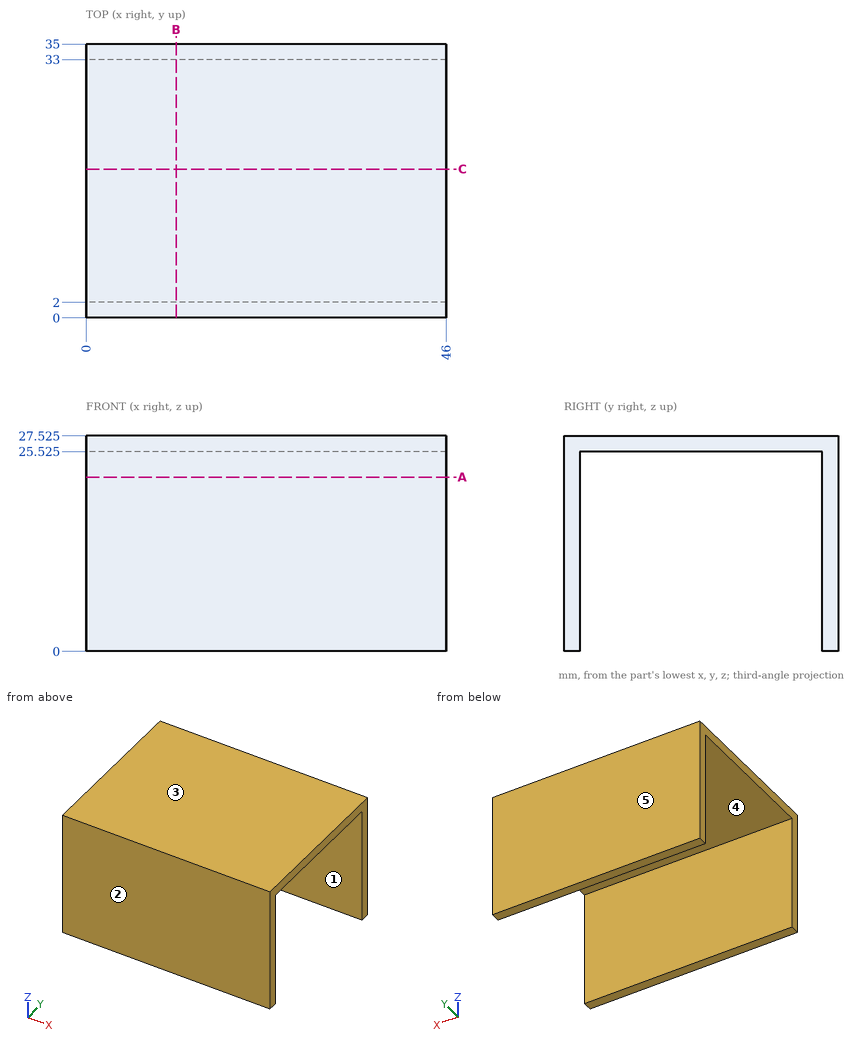
Job drawing, mm, ordinate dimensions from the low corner. One solid piece. A direction names the side the tool comes from. Give positions to 0.01 mm unless a question says otherwise; leave off trailing zeros. Write each loop counter-clockwise with the first axis right and the second up, starting at its lowest first coordinate (ties: lowest second). Pieces come first, ordered by that corner, then holes. Notation, with made-up numbers: M 50.25,51.5 L 93.25,51.5 A13 cw 93.25,71.5 Z; hole C 82.5,-25 d5. An arc over 180 degrees is marked long. One line per item, written item: value. Start each with the question number.
Q1. Probe probe 1 along Y at (x, z) = (15.5, 16); probe 2 along Z at (x, y) = (41, 19) (1 decimal). List the from-to ranges inside material, lowest first. Write a range as [from, to].
Q2. Saw through at C-C, the plane y = 19. Write the cut outline in (x, z) (1 decimal), plus the area to 3 significant figures.
Q3. Saw through at B-B, the plane x = 11.5. Write the cut outline in (y, z) (1 decimal), plus the area to 3 significant figures.
Q4. Two-plate mould, pull along Y, no slides. Class the marked faces 1, 2 and 3: +Y half, -Y half, draft (parallel to the pull), parting line (faces both ways), or undercut.
Q5. Saw through at A-A, the plane z = 22.25. Write the cut outline in (x, y), plus the area to 3 significant figures.
Q6. Drop a flat-ended pin along its axis: pin 1 Ø15.5 at (x, y) = (30.5, 24.5) entering from -Z (1 decimal). Give the stop position or say it passes through.
Q7. 3-axis set-ups, long thin cutter, end or side, ignore diameter. For the marked faces 4 and 5: which of +Z, -Z, +X, -X, +Y, -Y reach the whole face in a straight line?
Output values:
1. probe 1: y = [0, 2], [33, 35]
1. probe 2: z = [25.5, 27.5]
2. outline: M 0,25.5 L 46,25.5 L 46,27.5 L 0,27.5 Z
2. area: 92.0 mm²
3. outline: M 0,0 L 2,0 L 2,25.5 L 33,25.5 L 33,0 L 35,0 L 35,27.5 L 0,27.5 Z
3. area: 172 mm²
4. face 1: undercut
4. face 2: -Y half
4. face 3: draft
5. outline: M 0,0 L 46,0 L 46,2 L 0,2 Z; M 0,33 L 46,33 L 46,35 L 0,35 Z
5. area: 184 mm²
6. pin 1: stops at z = 25.5
7. face 4: -Z, +X, -X
7. face 5: +Z, -Z, +X, -X, +Y
